from build123d import *

# Parameters (mm, degrees)
BOSS_EXTRUDE1_DEPTH = 119
SKETCH2_W           = 15
SKETCH2_H           = 7
BOSS_EXTRUDE2_DEPTH = 9
SKETCH3_W           = 9
SKETCH3_H           = 7
CUT_EXTRUDE1_DEPTH  = 4
SKETCH4_W           = 5
SKETCH4_H           = 7
CUT_EXTRUDE2_DEPTH  = 12


with BuildPart() as part:
    # Sketch1 → Boss-Extrude1 (new body)
    with BuildSketch(Plane.XY):
        Polygon((-5.365984845, -2.186), (-7.365984845, -2.186), (-7.365984845, -3.186), (-4.365984845, -3.186), (-4.365984845, -2.186), (-4.365984845, 1.814), (4.634015155, 1.814), (4.634015155, -2.186), (4.634015155, -3.186), (7.634015155, -3.186), (7.634015155, -2.186), (5.634015155, -2.186), (5.634015155, 2.814), (-5.365984845, 2.814), align=None)
    extrude(amount=BOSS_EXTRUDE1_DEPTH)

    # Sketch2 → Boss-Extrude2 (add)
    with BuildSketch(Plane(origin=(0, -2.186, 0), x_dir=(1, 0, 0), z_dir=(0, 1, 0))):
        with Locations((0.134015155, -26.5)):
            Rectangle(SKETCH2_W, SKETCH2_H)
    extrude(amount=BOSS_EXTRUDE2_DEPTH)

    # Sketch3 → Cut-Extrude1 (cut)
    with BuildSketch(Plane.XZ.offset(2.186)):
        with Locations((0.134015155, 26.5)):
            Rectangle(SKETCH3_W, SKETCH3_H)
    extrude(amount=-CUT_EXTRUDE1_DEPTH, mode=Mode.SUBTRACT)

    # Sketch4 → Cut-Extrude2 (cut)
    with BuildSketch(Plane.ZY.offset(7.365984845)):
        with Locations((26.5, 2.314)):
            Rectangle(SKETCH4_W, SKETCH4_H)
    extrude(amount=-CUT_EXTRUDE2_DEPTH, mode=Mode.SUBTRACT)


solid = part.part
Read the model definition and answer for the solid it produces. Units are mm, in the model's axes. A direction names the side the tool comes from. Round coordinates to 2 decimals unless told otherwise and drop trailing zeros. Loops run counter-clockwise (first coordinate to the right, second up) from the corner with the lowest first, then second, coordinate; pieces in that order, holes last. Notation, with made-up numbers: (-23, 50.25) - (19, 50.25) arc R22 ccw to (19, 78.25) - close; hole circle Ø10 at (-5.75, -7.75). An arc over 180 degrees is marked (long way). One line per question, with ' | ' between items. Start each with the question number.
Q1. Section A-A on z = 27 is taken. Give the vertices of the cut face in (x, y), plus the area to 3 significant figures.
Q2. For faces 4 (the flat face through (-5.366, 0, 74)), 5 (the flat face through (5.634, 0, 11)), 6 (the flat face through (0, 1.814, 12)), 7 (the flat face through (-3, 3, 24)), 8 (the flat face through (7, -2.186, 74)), determine the directions among +Z, -Z, +X, -X, +Y, -Y from which every point of the face is accessible in a straight line to the end or side of a thin tool.
Q3. Flat-ended cylindrical pins translate along their axes: pin 1 (4 mm diameter, centred on x = -2, y = -1, fed in from -Z); pin 2 (5 mm diameter, centred on x = 3.5, y = -1.5, fed in from +Z); pin 3 (1.5 mm diameter, centred on y = 0.5, z = 72.5, fed in from +X); pin 4 (3 mm diameter, centred on y = 3, z = 19, fed in from -X). Find the tip coordinate at first contact, or state that the pin passes through.
Q4. Section D-D on z = 110 is taken. Give the vertices of the cut face in (x, y).
Q5. Section B-B on y = 0.5 is taken. Give the vertices of the cut face in (x, z), plus the area to 3 significant figures.
Q6. Find the intervals of material crossed by L1, parallel to X at y = -1, z = 72; L2, parallel to Z at x = -2.75, y = 4.25; L3, parallel to Z at x = -3.25, y = 2.5, in increasing order.
Q7. Section C-C on x = -1 is taken. Give the vertices of the cut face in (y, z), plus the area to 3 significant figures.
Q8. For a pull along Z with two mould halves and no side action, classify faces 1 (the flat face through (-6, -1.186, 26)), 2 (the flat face through (0, 2, 0)), 3 (the flat face through (0, 1.814, 73)) as +Z half, -Z half, draft (parallel to the pull), parting line (faces both ways), or undercut.
Established:
1) outline: (-7.37, -3.19) - (-4.37, -3.19) - (-4.37, -1.19) - (-7.37, -1.19) - close; (-7.37, 5.81) - (4.63, 5.81) - (4.63, -3.19) - (7.63, -3.19) - (7.63, 6.81) - (-7.37, 6.81) - close | area: 48.0 mm²
2) face 4: +Z, -X, +Y | face 5: -Z, +X, +Y | face 6: +Z, -Z, -Y | face 7: -X | face 8: +Z, +X, +Y
3) pin 1: through | pin 2: z = 119 | pin 3: x = 5.63 | pin 4: x = -5.37
4) outline: (-7.37, -3.19) - (-4.37, -3.19) - (-4.37, 1.81) - (4.63, 1.81) - (4.63, -3.19) - (7.63, -3.19) - (7.63, -2.19) - (5.63, -2.19) - (5.63, 2.81) - (-5.37, 2.81) - (-5.37, -2.19) - (-7.37, -2.19) - close
5) outline: (-7.37, 23) - (-5.37, 23) - (-5.37, 0) - (-4.37, 0) - (-4.37, 24) - (-7.37, 24) - close; (-7.37, 29) - (-4.37, 29) - (-4.37, 119) - (-5.37, 119) - (-5.37, 30) - (-7.37, 30) - close; (4.63, 0) - (5.63, 0) - (5.63, 23) - (7.63, 23) - (7.63, 30) - (5.63, 30) - (5.63, 119) - (4.63, 119) - close | area: 251 mm²
6) L1: -5.37 to -4.37, 4.63 to 5.63 | L2: 23 to 24, 29 to 30 | L3: 0 to 24, 29 to 119
7) outline: (1.81, 0) - (2.81, 0) - (2.81, 23) - (6.81, 23) - (6.81, 30) - (2.81, 30) - (2.81, 119) - (1.81, 119) - (1.81, 29) - (5.81, 29) - (5.81, 24) - (1.81, 24) - close | area: 127 mm²
8) face 1: undercut | face 2: -Z half | face 3: draft
